Design review of the part built by this model. Coordinates are the model's own, in mm. A direction names the side the tool comes from. Coordinates: 2 decimals unless noted, no trailing zeros. Loops run counter-clockwise (first coordinate to the right, second up) from the corner with the lowest first, then second, coordinate; pieces in that order, holes last. Notation, with made-up numbers: (5.25, 1) -> (25.25, 1) arc R30 cw to (25.25, 36) -> close; hole circle Ø8 at (63.5, 44). An arc over 180 degrees is marked (long way). One line per item, written item: value. Start each with the question number.
1. Insertion check: pin 1 (8 mm diameter, centred on x = 15.5, z = -51, fed in from +Y); pin 2 (4 mm diameter, centred on x = 29.5, z = -13, fed in from -Y); pin 3 (2.5 mm diameter, centred on y = 9.5, z = -45.5, fed in from +X). Each pin has a flat end and moves straight along its axis. Give the tip position at first contact, or say it passes through.
2. Machinability: for faces 4 (the flat face through (25, 5.7, -46)), 5 (the flat face through (48.17, 13.82, -45.39)), 6 (the cylindrical face through (7.77, -0.49, -86.1)), 7 (the conical face through (2.42, 10.28, -35.57)), which of the approach directions +Z, -Z, +X, -X, +Y, -Y give a long, thin tool a straight path to every point of the face, cutting with its end or side? Answer none if there is none.
3. For probe 1 along X at (y, z) = (9, -45.3); probe 2 along Z at (x, y) = (25.1, 10.75); probe 3 along Y at (x, z) = (25, -75), list the stretches that pass through material, from the lowest coordinate up.
4. Add section B-B on z = -83.4. Write out the cut boundary in (x, y).
5. Draft analysis for pull direction X (two halves, no side actions). For faces 1 (the flat face through (2.03, 6.88, -45.21)), 2 (the conical face through (47.78, 10.28, -55.03)), 3 (the cylindrical face through (33.64, 12.04, -28.89)), state which applies: pulls with the +X half, pulls with the -X half, needs draft (parallel to the pull), parting line crosses it, or undercut.
6. Add section C-C on y = 16.75. Write out the cut boundary in (x, z).
Autodesk Inventor part; units mm, degrees
ref_plane "Plano de trabajo1" through (25.1, 0, 0) normal (1, 0, 0) x (0, 0, -1)
ref_plane "YZ Plane" through (0, 0, 0) normal (1, 0, 0) x (0, 1, 0)
ref_plane "XZ Plane" through (0, 0, 0) normal (0, 1, 0) x (-1, 0, 0)
sketch "Boceto1" plane through (0, 0, 0) normal (0, 1, 0) x (-1, 0, 0)
  line L0 (0, 0) -> (-50.2, 0)
  line L1 (-50.2, 0) -> (-50.2, -90.6)
  line L2 (-50.2, -90.6) -> (0, -90.6)
  line L3 (0, -90.6) -> (0, 0)
  dimension "d0" = 50.2
  dimension "d1" = 90.6
extrude "Extrusión1" add sketch "Boceto1" along normal blind 20.7
sketch "Boceto2" plane through (0, 20.7, 0) normal (0, 1, 0) x (1, 0, 0)
  line L0 (-14.4985, 45.3) -> (58.2485, 45.3)
  circle A0 centre (25.1, 45.3) radius 18.5
  line L1 (50.2, 90.6) -> (0, 90.6)
  point P0 (0, 0)
  dimension "d7" = 37
  dimension "d51" = 90.6
  dimension "d52" = 0
extrude "Extrusión2" cut sketch "Boceto2" against normal blind 15
sketch "Boceto3" plane through (50.2, 0, 0) normal (1, 0, 0) x (0, 0, -1)
  line L0 (45.3, 28.8672) -> (45.3, -9.3744)
  line L1 (-5.2256, 10.35) -> (70.0589, 10.35)
  line L2 (38.65, 10.35) -> (51.95, 10.35) construction
  line L3 (38.65, 8.85) -> (51.95, 8.85)
  line L4 (51.95, 11.85) -> (38.65, 11.85)
  arc A0 (38.65, 11.85) -> (38.65, 8.85) centre (38.65, 10.35) ccw
  arc A1 (51.95, 8.85) -> (51.95, 11.85) centre (51.95, 10.35) ccw
  line L5 (90.6, 0) -> (90.6, 20.7)
  point P0 (0, 0)
  point P1 (45.3, 10.35)
  point P2 (53.45, 10.35)
  point P3 (37.15, 10.35)
  dimension "d11" = 16.3
  dimension "d12" = 3
  dimension "d13" = 0
  dimension "d53" = 45.3
extrude "Extrusión3" cut sketch "Boceto3" against normal blind 4
chamfer "Chaflán1" distance 4 angle 45 4 edges at (50.2, 8.85, -45.3) (50.2, 10.35, -37.15) (50.2, 11.85, -45.3) (50.2, 10.35, -53.45)
sketch "Boceto4" plane through (50.2, 0, 0) normal (1, 0, 0) x (0, 0, -1)
  point P0 (0, 0)
ref_plane "Plano de trabajo1" through (25.1, 0, 0) normal (1, 0, 0) x (0, 0, -1)
mirror "Simetría1" about plane through (25.1, 0, 0) normal (1, 0, 0) of "Extrusión3"
chamfer "Chaflán2" distance 4 angle 45 4 edges at (0, 11.85, -45.3) (0, 10.35, -37.15) (0, 8.85, -45.3) (0, 10.35, -53.45)
chamfer "Chaflán3" distance 2.5 angle 45 1 edges at (6.6, 20.7, -45.3)
sketch "Boceto5" plane through (0, 0, 0) normal (0, -1, 0) x (1, 0, 0)
  line L0 (25.1, 22.2035) -> (25.1, -86.3829)
  line L1 (-10.0483, -45.3) -> (59.9656, -45.3)
  circle A0 centre (6.05, -7.2) radius 3.2
  circle A1 centre (44.15, -7.2) radius 3.2
  circle A2 centre (44.15, -83.4) radius 3.2
  line L2 (0, 0) -> (50.2, 0)
  circle A3 centre (6.05, -83.4) radius 3.2
  dimension "d35" = 38.1
  dimension "d36" = 38.1
  dimension "d42" = 6.4
  dimension "d46" = 76.2
  dimension "d47" = 76.2
  dimension "d54" = 45.3
extrude "Extrusión4" add sketch "Boceto5" along normal blind 4.2
fillet "Empalme1" radius 3.2 4 edges at (40.95, -4.2, -7.2) (2.85, -4.2, -7.2) (40.95, -4.2, -83.4) (2.85, -4.2, -83.4)
properties material "Plastico PETG"
Worked answers:
1. pin 1: stops at y = 5.7
1. pin 2: stops at y = 0
1. pin 3: stops at x = 46.8
2. face 4: +Y
2. face 5: +X
2. face 6: -Y
2. face 7: -X
3. probe 1: x = 4 to 6.6, 43.6 to 46.2
3. probe 2: z = -90.6 to -63.8, -26.8 to 0
3. probe 3: y = 0 to 20.7
4. outline: (0, 0) -> (2.85, 0) -> (2.85, -1) arc R3.2 ccw to (9.25, -1) -> (9.25, 0) -> (40.95, 0) -> (40.95, -1) arc R3.2 ccw to (47.35, -1) -> (47.35, 0) -> (50.2, 0) -> (50.2, 20.7) -> (0, 20.7) -> close
5. face 1: pulls with the -X half
5. face 2: pulls with the +X half
5. face 3: undercut
6. outline: (0, -90.6) -> (50.2, -90.6) -> (50.2, 0) -> (0, 0) -> close; hole circle Ø37 at (25.1, -45.3)
